Part model, mm, in its own coordinate system. A direction names the side the tool comes from. Give positions to 0.01 mm unless a question says otherwise; leave off trailing zeros. Order: outer loops, then holes, each group sorted by start corner. A loop starts at its lowest first (then second) coordinate and runs counter-clockwise, first axis right, second up. Notation, with made-up numbers: (68, 86.5) - (73, 86.5) arc R26 ccw to (73, 121.5) - close; hole circle Ø7 at (80.5, 74.25). An arc over 180 degrees is marked (long way). One line per item, written item: value.
```python
from build123d import *

# Parameters (mm, degrees)
F0_R      = 42.8625
F1_DEPTH  = 38.1
F2_R      = 45.3625
F3_DEPTH  = 4
F4_R      = 40.3625
F5_DEPTH  = 5
F6_SIZE   = 1.5
F7_R      = 3.5
F8_DEPTH  = 2
F9_R      = 5
F10_DEPTH = 3
F12_DEPTH = 1.5
F13_SIZE  = 1
F14_R     = 1
F15_DEPTH = 5


with BuildPart() as f1:
    # F0 (on Top) → F1 (new body)
    with BuildSketch(Plane.XY):
        Circle(F0_R)
    extrude(amount=F1_DEPTH)

    # F2 (on face) → F3 (join)
    with BuildSketch(Plane.XY.offset(38.1)):
        Circle(F2_R)
    extrude(amount=F3_DEPTH)

    # F4 (on face) → F5 (cut)
    with BuildSketch(Plane.XY.offset(42.1)):
        Circle(F4_R)
    extrude(amount=-F5_DEPTH, mode=Mode.SUBTRACT)

    # F6
    f6_edges = [f1.edges().sort_by_distance(p)[0] for p in [
        (-45.3625, 0, 42.1),
        (-40.3625, 0, 42.1),
    ]]
    chamfer(f6_edges, length=F6_SIZE)

    # F7 (on face) → F8 (join)
    with BuildSketch(Plane.XY.offset(37.1)):
        Circle(F7_R)
    extrude(amount=F8_DEPTH)

    # F9 (on face) → F10 (join)
    with BuildSketch(Plane.XY.offset(39.1)):
        Circle(F9_R)
    extrude(amount=F10_DEPTH)

    # F11 (on face) → F12 (join)
    with BuildSketch(Plane.XY.offset(37.1)):
        Polygon((0, -3.5), (-3.5, 0), (-25.72323, -28.12019), align=None)
    extrude(amount=F12_DEPTH)

    # F13
    f13_edges = [f1.edges().sort_by_distance(p)[0] for p in [
        (-12.861615, -15.810095, 38.6),
        (-14.611615, -14.060095, 38.6),
    ]]
    chamfer(f13_edges, length=F13_SIZE)

    # F14 (on face) → F15 (join)
    with BuildSketch(Plane.XY.offset(37.1)):
        with Locations((-16, -23)):
            Circle(F14_R)
    extrude(amount=F15_DEPTH)


solid = f1.part
```
1) Slice it at A-A on z = 26.5. Write the cut outline in (x, y) (1 decimal), then the cut area to 3 significant figures.
Answer:
outline: circle Ø85.7 at (0, 0)
area: 5,770 mm2
2) Wall check: line 1 along Y through (x, z) = (0, 38.7); line 2 along Y through (x, z) = (0, 38); line 3 along Z through (x, y) = (35, -16). Give the ranges that are in metal, low to high. Write a range as [from, to].
Answer:
line 1: y = [-45.36, -40.36], [-3.5, 3.5], [40.36, 45.36]
line 2: y = [-42.86, -40.36], [-3.5, 3.5], [40.36, 42.86]
line 3: z = [0, 37.1]
3) Two-plate mould, pull along Z, no slides. Class faces 1 (the face through (39, -16, 42.1)), 2 (the face through (2.2, -3.3, 39.1)), 3 (the face through (37.285, -15.459, 38.874)), 4 (the face through (1.88, 2.95, 38.09)): pulls with the +Z half, pulls with the -Z half, needs draft (parallel to the pull), parting line crosses it, or undercut.
Answer:
face 1: pulls with the +Z half
face 2: undercut
face 3: needs draft
face 4: undercut
4) Which spindle directions (+Z, -Z, +X, -X, +Y, -Y) get a long thin tool onto all of the face, cutting with end or side? Do faces 5 (the face through (-1, 1, 0)), 6 (the face through (-7, -8, 38.6)), 7 (the face through (0, 0, 42.1)), 8 (the face through (-1.08, -4.88, 40.58)), 9 (the face through (40, -17, 38.1)). Say none if no direction does.
Answer:
face 5: -Z, +X, -X, +Y, -Y
face 6: none
face 7: +Z, +X, -X, +Y, -Y
face 8: +Z
face 9: -Z
5) Drop flat-ended pins along their axis: P1, Ø8, axis at x = 14, y = 18.5, coming from the +Z side; P2, Ø4.5, axis at x = -7.5, y = -7.5, coming from the +Z side; P3, Ø4, axis at y = 5.5, z = 18, coming from the +X side. Give the stop position or say it passes through.
Answer:
P1: stops at z = 37.1
P2: stops at z = 38.6
P3: stops at x = 42.72
